The listing builds one solid part. Answer for the finished solid, in the listing's coordinates (mm). Face numbers are marked on the shaded views. A direction names the side the tool comes from. Coordinates: 2 decimals unless noted, no trailing zeros. Write each loop counter-clockwise with the first axis right and the second up, starting at its lowest first coordinate (ties: lowest second). Pieces come first, ordered by that corner, then holes. Notation, with made-up numbers: M -22,0 L 17,0 A18 cw 17,4 Z; hole C -6,52.25 d8. An arc over 180 degrees is marked long. Answer as CSV lines item,"result". Start each with the question number.
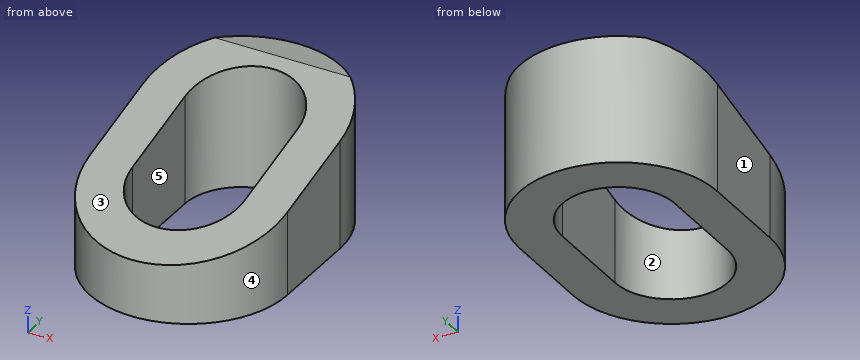
```python
from build123d import *

# Parameters (mm, degrees)
F1_DEPTH = 9
F5_W     = 42.8709182888
F5_H     = 32.7420830727
F6_DEPTH = 13


with BuildPart() as f1:
    # F0 (on Top) → F1 (new body)
    with BuildSketch(Plane.XY):
        with BuildLine():
            ThreePointArc((-6.9900002831, -3.26), (0, -10.2500002831), (6.9900002831, -3.26))
            Line((6.9900002831, -3.26), (6.9900002831, 0))
            Line((6.9900002831, 0), (6.9900002831, 3.26))
            ThreePointArc((6.9900002831, 3.26), (0, 10.2500002831), (-6.9900002831, 3.26))
            Line((-6.9900002831, 3.26), (-6.9900002831, 0))
            Line((-6.9900002831, 0), (-6.9900002831, -3.26))
        make_face()
        with BuildLine():
            ThreePointArc((-3.99, 3.26), (0, 7.25), (3.99, 3.26))
            Line((3.99, 3.26), (3.99, 0))
            Line((3.99, 0), (3.99, -3.26))
            ThreePointArc((3.99, -3.26), (0, -7.25), (-3.99, -3.26))
            Line((-3.99, -3.26), (-3.99, 0))
            Line((-3.99, 0), (-3.99, 3.26))
        make_face(mode=Mode.SUBTRACT)
    extrude(amount=F1_DEPTH)

    # F5 (on offset) → F6 (cut)
    with BuildSketch(Plane(origin=(0, -5.0565690429, 18.8713725799), x_dir=(1, 0, 0), z_dir=(0, -0.2588190451, 0.9659258263))):
        with Locations((-1.5699611977, 4.9039889127)):
            Rectangle(F5_W, F5_H)
    extrude(amount=-F6_DEPTH, mode=Mode.SUBTRACT)


solid = f1.part
```
1) Which of the six approach directions +Z, -Z, +X, -X, +Y, -Y give full straight-line access (tool end or side, diameter ignored) to the marked faces 4 and 5?
2) Find the intervals of material crossed by line 1 (X direction, y = 6.25, z = 1.5); line 2 (Y direction, x = 0, z = 5.25); line 3 (X direction, y = -4, z = 3.5), in increasing order. Write a range as from..to.
3) Each of these flat-tipped pins is pushed along its axis until it touches: P1, Ø4, axis at x = -3.5, z = 1.5, coming from the -Y side; P2, Ø2, axis at x = 3.5, y = 1, coming from the +Z side; P3, Ø4, axis at x = 2, y = -6, coming from the +Z side. Where does it stop, or does it pass through?
4) The part is cut by section B-B (y = -3.5). Determine the outline of the cut face in (x, z).
5) For a pull along X with two mould halves and no side action, classify the marked faces 1, 2 and 3 as +X half, -X half, draft (parallel to the pull), parting line (faces both ways), or undercut.
6) The part is cut by section A-A (x = -1). Determine the outline of the cut face in (y, z).
7) The part is cut by section C-C (z = 1.75). Determine the outline of the cut face in (x, y), then the cut area to 3 significant figures.
8) The part is cut by section D-D (x = 3.75). Determine the outline of the cut face in (y, z), then the cut area to 3 significant figures.
Completed:
1,face 4,"+Z, -Z, -Y"
1,face 5,"+Z, -Z"
2,line 1,"-6.32..-2.64, 2.64..6.32"
2,line 2,"7.25..10.25"
2,line 3,"-6.95..-3.92, 3.92..6.95"
3,P1,"y = -10.09"
3,P2,"z = 7.27"
3,P3,"z = 5.46"
4,outline,"M -6.99,0 L -3.98,0 L -3.98,5.83 L -6.99,5.83 Z; M 3.98,0 L 6.99,0 L 6.99,5.83 L 3.98,5.83 Z"
5,face 1,"-X half"
5,face 2,"undercut"
5,face 3,"draft"
6,outline,"M -10.18,0 L -7.12,0 L -7.12,4.86 L -10.18,4.04 Z; M 7.12,0 L 10.18,0 L 10.18,9 L 8.33,9 L 7.12,8.68 Z"
7,outline,"M -6.99,-3.26 A6.99 ccw 6.99,-3.26 L 6.99,3.26 A6.99 ccw -6.99,3.26 Z; hole M -3.99,-3.26 A3.99 ccw 3.99,-3.26 L 3.99,3.26 A3.99 ccw -3.99,3.26 Z"
7,area,"143 mm²"
8,outline,"M -9.16,0 L -4.62,0 L -4.62,5.53 L -9.16,4.31 Z; M 4.62,0 L 9.16,0 L 9.16,9 L 8.33,9 L 4.62,8.01 Z"
8,area,"61.3 mm²"
